Design review of the part built by this model. Coordinates are the model's own, in mm. A direction names the side the tool comes from. Give positions to 0.01 mm unless a question says otherwise; leave off trailing zeros. Loops run counter-clockwise (first coordinate to the right, second up) from the corner with the lowest first, then second, coordinate; pieces in that order, holes last. Notation, with made-up numbers: M 22.25,73 L 71.25,73 A13 ccw 71.25,88 Z; hole C 81.5,-14.5 d9. An arc over 180 degrees is marked long. Answer as CSV lines item,"result".
```python
from build123d import *

# Parameters (mm, degrees)
SKETCH_1_W          = 100
SKETCH_1_H          = 50
SKETCH_1_R          = 1.7
EXTRUDE_1_DEPTH     = 5
HOLE_WIZARD_M2_2_D  = 1.6
SKETCH_8_R          = 8
SKETCH_8_R_2        = 6
EXTRUDE_1_2_DEPTH   = 60
CUT_EXTRUDE_START   = -60
CUT_EXTRUDE_1_DEPTH = 60


with BuildPart() as part:
    # 草图1 → Extrude 1 (new body)
    # profile 1 of 3: a face of its own
    with BuildSketch(Plane(origin=(0, 0, 0), x_dir=(1, 0, 0), z_dir=(0, 1, 0))):
        Rectangle(SKETCH_1_W, SKETCH_1_H)
        with Locations(Location((-45, -20, 0), (0, 0, 270))):
            Circle(SKETCH_1_R, mode=Mode.SUBTRACT)
        with Locations(Location((45, -20, 0), (0, 0, 270))):
            Circle(SKETCH_1_R, mode=Mode.SUBTRACT)
        with Locations(Location((-45, 20, 0), (0, 0, 270))):
            Circle(SKETCH_1_R, mode=Mode.SUBTRACT)
        with Locations(Location((45, 20, 0), (0, 0, 270))):
            Circle(SKETCH_1_R, mode=Mode.SUBTRACT)
    # profile 2 of 3: a face of its own
    with BuildSketch(Plane(origin=(0, 0, 0), x_dir=(1, 0, 0), z_dir=(0, 1, 0))):
        with BuildLine():
            Line((-50, 25), (-85, 25))
            ThreePointArc((-85, 25), (-88.535533906, 23.535533906), (-90, 20))
            Line((-90, 20), (-90, -20))
            ThreePointArc((-90, -20), (-88.535533906, -23.535533906), (-85, -25))
            Line((-85, -25), (-50, -25))
            Line((-50, -25), (-50, 25))
        make_face()
        with Locations(Location((-85, -20, 0), (0, 0, 270))):
            Circle(SKETCH_1_R, mode=Mode.SUBTRACT)
        with Locations(Location((-85, 20, 0), (0, 0, 270))):
            Circle(SKETCH_1_R, mode=Mode.SUBTRACT)
    # profile 3 of 3: a face of its own
    with BuildSketch(Plane(origin=(0, 0, 0), x_dir=(1, 0, 0), z_dir=(0, 1, 0))):
        with BuildLine():
            Line((85, 25), (50, 25))
            Line((50, 25), (50, -25))
            Line((50, -25), (85, -25))
            ThreePointArc((85, -25), (88.535533906, -23.535533906), (90, -20))
            Line((90, -20), (90, 20))
            ThreePointArc((90, 20), (88.535533906, 23.535533906), (85, 25))
        make_face()
        with Locations(Location((85, -20, 0), (0, 0, 270))):
            Circle(SKETCH_1_R, mode=Mode.SUBTRACT)
        with Locations(Location((85, 20, 0), (0, 0, 270))):
            Circle(SKETCH_1_R, mode=Mode.SUBTRACT)
    extrude(amount=EXTRUDE_1_DEPTH)

    # M2 螺纹孔2 (through all)
    with Locations(Plane(origin=(0, 5, 0), x_dir=(1, 0, 0), z_dir=(0, 1, 0))):
        with Locations((-7.5, 19), (7.5, 19)):
            Hole(HOLE_WIZARD_M2_2_D / 2)

    # 草图8 → Extrude 1 2 (add)
    with BuildSketch(Plane(origin=(0, 5, 0), x_dir=(1, 0, 0), z_dir=(0, 1, 0))):
        with Locations((-80, 0)):
            Circle(SKETCH_8_R)
        with Locations((-80, 0)):
            Circle(SKETCH_8_R_2, mode=Mode.SUBTRACT)
    extrude(amount=EXTRUDE_1_2_DEPTH)

    # 草图9 → 切除-拉伸1 (cut)
    with BuildSketch(Plane(origin=(0, 65, 0), x_dir=(1, 0, 0), z_dir=(0, 1, 0)).offset(CUT_EXTRUDE_START)):
        with BuildLine():
            Line((-74.190524981, 1.5), (-72.141883177, 1.5))
            ThreePointArc((-72.141883177, 1.5), (-72, 0), (-72.141883177, -1.5))
            Line((-72.141883177, -1.5), (-74.190524981, -1.5))
            ThreePointArc((-74.190524981, -1.5), (-74, 0), (-74.190524981, 1.5))
        make_face()
    extrude(amount=CUT_EXTRUDE_1_DEPTH, mode=Mode.SUBTRACT)


solid = part.part
```
1. The part is to be moulded in two halves that separate along Z. For faces 1 (the flat face through (-90, 2, 0)), 2 (the cylindrical face through (-89, 2, 23)), 3 (the cylindrical face through (-86.5, 2.5, 20.8)), say which applies: pulls with the +Z half, pulls with the -Z half, needs draft (parallel to the pull), parting line crosses it, or undercut.
Answer block:
face 1,"needs draft"
face 2,"pulls with the +Z half"
face 3,"undercut"
2. We need section D-D, the plane x = -77.5. Write out the cut boundary in (y, z), plus the area to 3 significant figures.
Answer block:
outline,"M 0,-25 L 5,-25 L 5,-7.6 L 65,-7.6 L 65,-5.45 L 5,-5.45 L 5,5.45 L 65,5.45 L 65,7.6 L 5,7.6 L 5,25 L 0,25 Z"
area,"507 mm²"
3. For P1, Ø12, axis at y = 27, z = -15, coming from the +X side; P2, Ø10, axis at x = -3, z = -11, coming from the +Y side; P3, Ø0.6, axis at x = -73, y = 36, coming from the -Z side; P4, Ø5, axis at y = 54, z = 9.5, coming from the -X side, all flat-tipped, find the tip position at first contact; note any pin that passes through.
Answer block:
P1,"through"
P2,"y = 5"
P3,"z = -4.37"
P4,"x = -83.87"
4. For faces 4 (the flat face through (90, 2, 0)), 5 (the cylindrical face through (-86, 35, 0)), list the 3-axis set-ups (+Z, -Z, +X, -X, +Y, -Y) from which the entire face can be reached by the end or side of a thin tool; tool diameter is ignored.
Answer block:
face 4,"+Z, -Z, +X, +Y, -Y"
face 5,"+Y"
5. To check wall thickness, follow L1, parallel to X at y = 1.35, z = -20; L2, parallel to Z at x = -85, y = 2.75; L3, parallel to Z at x = -80, y = 50.5. State the ranges of each line that lie inside material, in increasing order. Write a range as [from, to].
Answer block:
L1,"[-90, -86.7], [-83.3, -46.7], [-43.3, 43.3], [46.7, 83.3], [86.7, 90]"
L2,"[-25, -21.7], [-18.3, 18.3], [21.7, 25]"
L3,"[-8, -6], [6, 8]"
6. We need section B-B, the plane y = 45. Write out the cut boundary in (x, z), plus the area to 3 significant figures.
Answer block:
outline,"M -74.19,-1.5 A6 cw long -74.19,1.5 L -72.14,1.5 A8 ccw long -72.14,-1.5 Z"
area,"81.9 mm²"
7. We need section A-A, the plane x = 45. Write out the cut boundary in (y, z).
Answer block:
outline,"M 0,-25 L 5,-25 L 5,-21.7 L 0,-21.7 Z; M 0,-18.3 L 5,-18.3 L 5,18.3 L 0,18.3 Z; M 0,21.7 L 5,21.7 L 5,25 L 0,25 Z"
8. We need section C-C, the plane x = 76.5. Write out the cut boundary in (y, z), plus the area to 3 significant figures.
Answer block:
outline,"M 0,-25 L 5,-25 L 5,25 L 0,25 Z"
area,"250 mm²"
